```python
from build123d import *

# Parameters (mm, degrees)
BOSS_EXTRUDE1_DEPTH = 12
SKETCH2_R           = 2
CUT_EXTRUDE1_DEPTH  = 20


with BuildPart() as part:
    # Sketch1 → Boss-Extrude1 (new body)
    with BuildSketch(Plane.XY):
        with BuildLine():
            Line((27, 10.648423286), (27, 15))
            ThreePointArc((27, 15), (31.017062028, 14.31079961), (35.086282243, 14.08008038))
            Line((35.086282243, 14.08008038), (35.086282243, 24.18008038))
            ThreePointArc((35.086282243, 24.18008038), (9.186282243, 50.08008038), (35.086282243, 75.98008038))
            Line((35.086282243, 75.98008038), (35.086282243, 90.332329282))
            ThreePointArc((35.086282243, 90.332329282), (-4.960293251, 54.143986489), (27, 10.648423286))
        make_face()
    extrude(amount=BOSS_EXTRUDE1_DEPTH)

    # Sketch2 → Cut-Extrude1 (cut)
    with BuildSketch(Plane.XY.offset(12)):
        with Locations((10.086282243, 74.574977808)):
            Circle(SKETCH2_R)
        with Locations((11.117766586, 24.574977808)):
            Circle(SKETCH2_R)
    extrude(amount=-CUT_EXTRUDE1_DEPTH, mode=Mode.SUBTRACT)


solid = part.part
```
Geometry: final body of the model. Coordinates: model frame, mm. A direction names the side the tool comes from. Round coordinates to 2 decimals unless told otherwise and drop trailing zeros. Write each loop counter-clockwise with the first axis right and the second up, starting at its lowest first coordinate (ties: lowest second). Pieces come first, ordered by that corner, then holes. Notation, with made-up numbers: M 8.5,-4.5 L 63.5,-4.5 A25 cw 63.5,23.5 Z; hole C 44.5,81 d3. An arc over 180 degrees is marked long. Answer in a Markdown table with one row per item. Add a question column.
(1) Cut plane C-C, the plane y = 44. Return the cut outline in (x, z).
(2) Draft query along Y for faces 1 (the face through (9.644, 25.927, 6.084)), 2 (the face through (9.193, 49.511, 5.916)), 3 (the face through (-4.868, 54.967, 5.916)), 4 (the face through (6, 51, 0)). Return one class per face: pulls with the +Y half, pulls with the -Y half, needs draft (parallel to the pull), parting line crosses it, or undercut.
(3) Cut plane A-A, the plane x = 26. Return the cut outline in (y, z), then the cut area to 3 significant figures.
(4) Ray query, L1, parallel to Y at x = 15, z = 9.75; L2, parallel to Y at x = 22.5, z = 5.5; L3, parallel to X at y = 65.5, z = 1.5. Return the intervals inside material, ascending.
(5) Cut plane B-B, the plane z = 6.75. Return the cut outline in (x, y).
(6) Cut plane D-D, the plane x = -2. Return the cut outline in (y, z).
(7) Contact query for flat-ended pins moving along their axis: pin 1 (2 mm diameter, centred on x = 0.5, z = 6, fed in from -Y); pin 2 (1.5 mm diameter, centred on y = 49, z = 3.5, fed in from -X); pin 3 (2.5 mm diameter, centred on x = 10.09, y = 74.57, fed in from -Z); pin 4 (5 mm diameter, centred on x = 14.5, z = 9, fed in from +Y). Output: stop coordinate, or through.
(8) Reachability of faces 5 (the face through (9.83, 76.56, 6.08)), 6 (the face through (27, 13, 6)) from +Z, -Z, +X, -X, +Y, -Y: full face, straight path, thin tool, end or side. Return the list, or none.
Established:
| question | item | result |
|---|---|---|
| 1 | outline | M -4.7,0 L 9.91,0 L 9.91,12 L -4.7,12 Z |
| 2 | face 1 | undercut |
| 2 | face 2 | undercut |
| 2 | face 3 | parting line crosses it |
| 2 | face 4 | needs draft |
| 3 | outline | M 10.87,0 L 25.83,0 L 25.83,12 L 10.87,12 Z; M 74.33,0 L 89.29,0 L 89.29,12 L 74.33,12 Z |
| 3 | area | 359 mm² |
| 4 | L1 | 15.2 to 33.73, 66.43 to 84.96 |
| 4 | L2 | 11.85 to 27.44, 72.72 to 88.31 |
| 4 | L3 | -2.1 to 14.28 |
| 5 | outline | M 27,10.65 L 27,15 A36 ccw 35.09,14.08 L 35.09,24.18 A25.9 cw 35.09,75.98 L 35.09,90.33 A40.25 ccw Z; hole C 10.09,74.57 d4; hole C 11.12,24.57 d4 |
| 6 | outline | M 34.43,0 L 65.73,0 L 65.73,12 L 34.43,12 Z |
| 7 | pin 1 | y = 27.89 |
| 7 | pin 2 | x = -5.16 |
| 7 | pin 3 | through |
| 7 | pin 4 | y = 86.04 |
| 8 | face 5 | +Z, -Z |
| 8 | face 6 | +Z, -Z, -Y |
